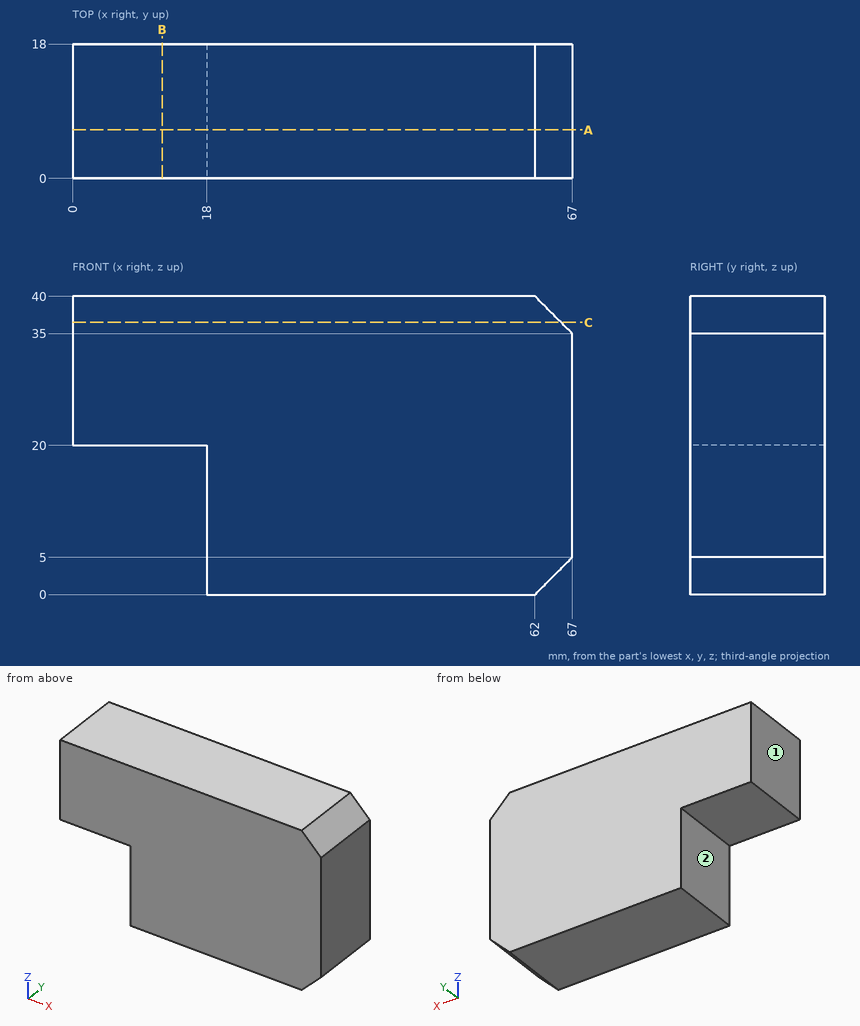
Can you work these out from the drawing? Everything is in mm from the part's minimum corner. A direction names the side the tool comes from. Coordinates: 2 decimals unless noted, no trailing zeros. Loops run counter-clockwise (first coordinate to the right, second up) from the corner with the lowest first, then second, coordinate; pieces in that order, holes last. Notation, with made-up numbers: (51, 52) - (106, 52) arc R23 cw to (106, 89) - close; hole circle Ø9 at (30, 7). An arc over 180 degrees is marked (long way). Answer as CSV lines item,"result".
Q1. If we section it at C-C, the plane z = 36.5: Write out the boundary of the cut face in (x, y), and give its area (3 significant figures).
Response:
outline,"(0, 0) - (65.5, 0) - (65.5, 18) - (0, 18) - close"
area,"1,180 mm2"
Q2. For the marked faces 1 and 2, which set-ups out of +Z, -Z, +X, -X, +Y, -Y let a thin tool reach every point of the face, with its end or its side?
Response:
face 1,"+Z, -Z, -X, +Y, -Y"
face 2,"-Z, -X, +Y, -Y"
Q3. If we section it at B-B, the plane x = 12: Write out the boundary of the cut face in (y, z).
Response:
outline,"(0, 20) - (18, 20) - (18, 40) - (0, 40) - close"
Q4. If we section it at A-A, the plane y = 6.5: Write out the boundary of the cut face in (x, z).
Response:
outline,"(0, 20) - (18, 20) - (18, 0) - (62, 0) - (67, 5) - (67, 35) - (62, 40) - (0, 40) - close"
Q5. If I drill on L1, parallel to X at y = 15.75, z = 9.5; L2, parallel to Z at x = 7, y = 2; L3, parallel to X at y = 6.75, z = 35.5, over which ranges is the centre line in solid material (lowest first)? Write a range as [from, to].
Response:
L1,"[18, 67]"
L2,"[20, 40]"
L3,"[0, 66.5]"
Q6. For pin 1 (10 mm diameter, centred on y = 8, z = 11, fed in from -X); pin 2 (5.5 mm diameter, centred on x = 12, y = 7, fed in from -Z), each with a flat end and sliding along its axis, tell me the tip position at first contact or that it passes through.
Response:
pin 1,"x = 18"
pin 2,"z = 20"
